Can you work these out from the model? Positions are in its coordinate system, mm. A direction names the side the tool comes from. Round coordinates to 2 decimals unless told otherwise and drop trailing zeros. Loops run counter-clockwise (first coordinate to the right, second up) from the corner with the lowest first, then second, coordinate; pieces in that order, holes last.
from build123d import *

# Parameters (mm, degrees)
F0_R     = 3
F1_DEPTH = 3.95
F0_R_2   = 2.499
F0_R_3   = 2.495
F2_DEPTH = 3.45
F3_R     = 3.69999
F4_R     = 3.69999


# Not quite as in the source:
# - a fillet or chamfer is up to 0.001 mm smaller than in the source, because OpenCascade refuses the exact size


with BuildPart() as f1:
    # F0 (on Front) → F1 (new body, symmetric)
    with BuildSketch(Plane.XZ):
        Polygon((-39.65, 3.7), (-39.65, -3.7), (39.65, -3.7), (39.65, 3.7), (0, 3.7), align=None)
        with Locations((-36, 0)):
            Circle(F0_R, mode=Mode.SUBTRACT)
        with Locations((-28, 0)):
            Circle(F0_R, mode=Mode.SUBTRACT)
        with Locations((-20, 0)):
            Circle(F0_R, mode=Mode.SUBTRACT)
        with Locations((-12, 0)):
            Circle(F0_R, mode=Mode.SUBTRACT)
        with Locations((-4, 0)):
            Circle(F0_R, mode=Mode.SUBTRACT)
        with BuildLine():
            ThreePointArc((7, 0), (4, -3), (1, 0))
            ThreePointArc((1, 0), (4, 3), (7, 0))
        make_face(mode=Mode.SUBTRACT)
        with Locations((12, 0)):
            Circle(F0_R, mode=Mode.SUBTRACT)
        with Locations((20, 0)):
            Circle(F0_R, mode=Mode.SUBTRACT)
        with Locations((28, 0)):
            Circle(F0_R, mode=Mode.SUBTRACT)
        with Locations((36, 0)):
            Circle(F0_R, mode=Mode.SUBTRACT)
    extrude(amount=F1_DEPTH, both=True)

    # F0 (on Front) → F2 (join, symmetric)
    with BuildSketch(Plane.XZ):
        with Locations((-36, 0)):
            Circle(F0_R)
        with Locations((-36, 0)):
            Circle(F0_R_2, mode=Mode.SUBTRACT)
        with Locations((-28, 0)):
            Circle(F0_R)
        with Locations((-28, 0)):
            Circle(F0_R_2, mode=Mode.SUBTRACT)
        with Locations((-20, 0)):
            Circle(F0_R)
        with Locations((-20, 0)):
            Circle(F0_R_2, mode=Mode.SUBTRACT)
        with Locations((-12, 0)):
            Circle(F0_R)
        with Locations((-12, 0)):
            Circle(F0_R_2, mode=Mode.SUBTRACT)
        with Locations((-4, 0)):
            Circle(F0_R)
        with Locations((-4, 0)):
            Circle(F0_R_2, mode=Mode.SUBTRACT)
        with BuildLine():
            ThreePointArc((7, 0), (4, 3), (1, 0))
            ThreePointArc((1, 0), (4, -3), (7, 0))
        make_face()
        with BuildLine():
            ThreePointArc((6.499, 0), (4, -2.499), (1.501, 0))
            ThreePointArc((1.501, 0), (4, 2.499), (6.499, 0))
        make_face(mode=Mode.SUBTRACT)
        with Locations((12, 0)):
            Circle(F0_R)
        with Locations((12, 0)):
            Circle(F0_R_3, mode=Mode.SUBTRACT)
        with Locations((20, 0)):
            Circle(F0_R)
        with Locations((20, 0)):
            Circle(F0_R_2, mode=Mode.SUBTRACT)
        with Locations((28, 0)):
            Circle(F0_R)
        with Locations((28, 0)):
            Circle(F0_R_2, mode=Mode.SUBTRACT)
        with Locations((36, 0)):
            Circle(F0_R)
        with Locations((36, 0)):
            Circle(F0_R_2, mode=Mode.SUBTRACT)
    extrude(amount=F2_DEPTH, both=True)

    # F3 (radius 3.7 in the source; OpenCascade refuses exactly that, so slightly less here)
    f3_edges = [f1.edges().sort_by_distance(p)[0] for p in [
        (39.65, 0, 3.7),
        (39.65, 0, -3.7),
    ]]
    fillet(f3_edges, radius=F3_R)

    # F4 (radius 3.7 in the source; OpenCascade refuses exactly that, so slightly less here)
    f4_edges = [f1.edges().sort_by_distance(p)[0] for p in [
        (-39.65, 0, 3.7),
        (-39.65, 0, -3.7),
    ]]
    fillet(f4_edges, radius=F4_R)


solid = f1.part
(1) Will this pin go through, and if not, where does the flat tip stop? P1, Ø1.5, axis at y = -2.5, z = 1.5, coming from the -X side.
Worked answers:
P1: stops at x = -39.57
(2) If we mould it in two halves opening along X, with no side actions, what happens to faces 4 (the flat face through (-0.6, -3.95, 0.1)), 5 (the cylindrical face through (38.59, 0.06, 2.59)), 6 (the cylindrical face through (-38.54, -0.06, -2.64)), 7 (the cylindrical face through (-25.616, 0.048, 0.751))? For each: released by +X, released by -X, zero draft, split by the parting line, or undercut.
Worked answers:
face 4: zero draft
face 5: released by +X
face 6: released by -X
face 7: undercut
(3) If we section it at B-B, the plane y = 1.5: State how many separate pieces and enclosed holes the cut face has, then the cut area to 3 significant figures.
Worked answers:
separate pieces: 1
enclosed holes: 10
area: 379 mm2
(4) If we section it at A-A, the plane x = 28: List the corners of the cut face in (y, z) for me.
Worked answers:
outline: (-3.95, -3.7) - (3.95, -3.7) - (3.95, -3) - (3.45, -3) - (3.45, -2.5) - (-3.45, -2.5) - (-3.45, -3) - (-3.95, -3) - close; (-3.95, 3) - (-3.45, 3) - (-3.45, 2.5) - (3.45, 2.5) - (3.45, 3) - (3.95, 3) - (3.95, 3.7) - (-3.95, 3.7) - close
(5) For faces 1 (the cylindrical face through (-1.14, 3.7, 0.9)), 2 (the cylindrical face through (-17.616, 0.048, 0.751)), 3 (the cylindrical face through (25, -3.7, 0.1)), which set-ups out of +Z, -Z, +X, -X, +Y, -Y let a thin tool reach every point of the face, with its end or its side?
Worked answers:
face 1: +Y
face 2: +Y, -Y
face 3: -Y
(6) If we section it at C-C, the plane x = -28.5: List the corners of the cut face in (y, z) for me.
Worked answers:
outline: (-3.95, -3.7) - (3.95, -3.7) - (3.95, -2.96) - (3.45, -2.96) - (3.45, -2.45) - (-3.45, -2.45) - (-3.45, -2.96) - (-3.95, -2.96) - close; (-3.95, 2.96) - (-3.45, 2.96) - (-3.45, 2.45) - (3.45, 2.45) - (3.45, 2.96) - (3.95, 2.96) - (3.95, 3.7) - (-3.95, 3.7) - close
(7) If I drill on line 1 (Z direction, x = -18, y = -0.75); line 2 (Z direction, x = -4, y = -3.8); line 3 (Y direction, x = 35.5, z = 2.5), over which ranges is the centre line in solid material (lowest first)?
Worked answers:
line 1: z = -3.7 to -1.5, 1.5 to 3.7
line 2: z = -3.7 to -3, 3 to 3.7
line 3: y = -3.45 to 3.45
